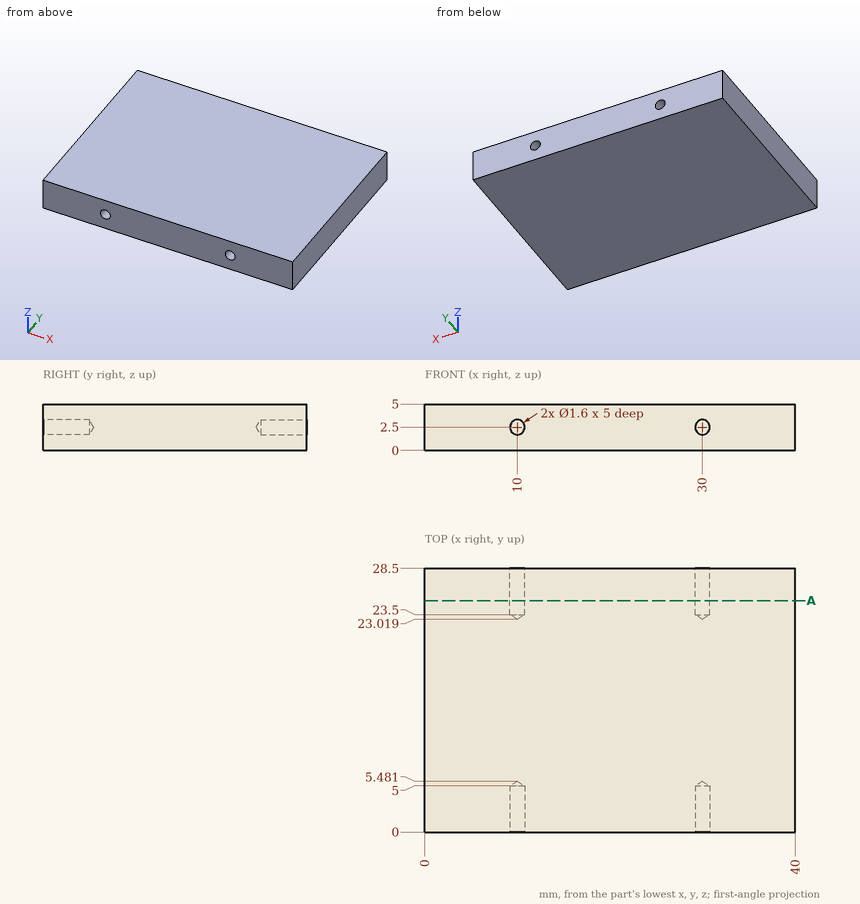
Input: dimensioned drawing with shaded views. Units: mm. Origin: part minimum x, y, z. Give positions to 0.01 mm unless a question says otherwise; leave off trailing zeros. Order: outer loops, then holes, each group sorted by start corner. A loop starts at its lowest first (then second) coordinate and runs counter-clockwise, first axis right, second up. Notation, with made-up numbers: (63.25, 12) -> (122.25, 12) arc R7 ccw to (122.25, 18) -> close; hole circle Ø10 at (34.25, -2). An arc over 180 degrees is marked (long way). Answer as a JSON object with one key per item and string values.
Q1. Section A-A (y = 25). Output: boundary loops of the cut face in (x, z), plus the area to 3 significant figures.
Entries:
{"outline": "(0, 0) -> (40, 0) -> (40, 5) -> (0, 5) -> close; hole circle Ø1.6 at (10, 2.5); hole circle Ø1.6 at (30, 2.5)", "area": "196 mm^2"}
Q2. Material intervals for probe 1 along X at (y, z) = (25.45, 2.5); probe 2 along Z at (x, y) = (10, 24.8), sorted ascending.
Entries:
{"probe 1": "x = 0 to 9.2, 10.8 to 29.2, 30.8 to 40", "probe 2": "z = 0 to 1.7, 3.3 to 5"}
Q3. First-contact query: pin 1 (1.3 mm diameter, centred on x = 30, z = 2.5, fed in from -Y); pin 2 (5 mm diameter, centred on x = 14.5, y = 18, fed in from -Z); pin 3 (1.4 mm diameter, centred on x = 10, z = 2.5, fed in from +Y). Flat tips, straight axial feed; report the tip coordinate or a pass-through.
Entries:
{"pin 1": "stops at y = 5.09", "pin 2": "stops at z = 0", "pin 3": "stops at y = 23.44"}
